Geometry: final body of the model. Coordinates: model frame, mm. A direction names the side the tool comes from. Coordinates: 2 decimals unless noted, no trailing zeros. Write each loop counter-clockwise with the first axis right and the second up, starting at its lowest first coordinate (ties: lowest second). Pieces come first, ordered by that corner, then holes. Notation, with made-up numbers: (57.5, -29.5) - (70.5, -29.5) arc R22 cw to (70.5, -0.5) - close; hole circle Ø1 at (82, 19). An arc over 180 degrees is marked (long way). Answer as a JSON object with one key per item and string values. Group by question number.
Item 1: Line query: line 1 along Y through (x, z) = (25.5, 2.75); line 2 along Y through (x, z) = (51, 6); line 3 along X through (y, z) = (-9, 2.75). Output: solid intervals per line, ascending. Write a range as from..to.
Item 2: Mould query, pull axis X, two halves, no side actions, for faces 5 (the flat face through (7, 46.373, 1)), 6 (the flat face through (73.128, 3, 2)), 7 (the flat face through (2, -44, 0)), 8 (the flat face through (9, -47.627, 5)). Classes: pulls with the +X half, pulls with the -X half, needs draft (parallel to the pull), parting line crosses it, or undercut.
Item 3: First-contact query: pin 1 Ø8 at (x, y) = (54, -39) entering from +Z; pin 2 Ø3 at (y, z) = (5, 5.5) entering from +X. Flat tips, straight axial feed; report the tip coordinate or a pass-through.
Item 4: Set-up query: faces 1 (the flat face through (7, 54.373, 3)), 2 (the flat face through (71.128, -45, 5)), 3 (the flat face through (8, 52.373, 5)), 4 (the flat face through (8, -41.627, 1)). Return all of +Z, -Z, +X, -X, +Y, -Y with unobstructed straight access to the full face (end or side cutting, diameter ignored); none if empty.
Item 5: Section A-A on y = 25.5. Return loops of the section in (x, z).
Item 6: Section B-B on x = 18. Return loops of the section in (y, z).
Item 7: Section C-C on z = 1.25. Return loops of the section in (x, y), and give its area (3 significant figures).
Autodesk Fusion 360 part; units mm, degrees
sketch "Sketch2" plane through (0, 0, 0) normal (0, 0, 1) x (1, 0, 0)
  line L0 (-55.8718, 52.373) -> (71.1282, 52.373)
  line L1 (71.1282, 52.373) -> (71.1282, -47.627)
  line L2 (71.1282, -47.627) -> (-55.8718, -47.627)
  line L3 (-55.8718, -47.627) -> (-55.8718, 52.373)
  line L4 (-51.3718, 46.373) -> (66.6282, 46.373)
  line L5 (66.6282, 46.373) -> (66.6282, -41.627)
  line L6 (66.6282, -41.627) -> (-51.3718, -41.627)
  line L7 (-51.3718, -41.627) -> (-51.3718, 46.373)
  line L8 (-57.8718, 54.373) -> (73.1282, 54.373)
  line L9 (73.1282, 54.373) -> (73.1282, -49.627)
  line L10 (73.1282, -49.627) -> (-57.8718, -49.627)
  line L11 (-57.8718, -49.627) -> (-57.8718, 54.373)
  dimension "d1" = 127
  dimension "d2" = 100
  dimension "d3" = 118
  dimension "d4" = 88
  dimension "d5" = 131
  dimension "d6" = 104
  dimension "d7" = 2
  dimension "d8" = 2
  dimension "d43" = 4.5
  dimension "d44" = 6
extrude "Extrude7" add sketch "Sketch2" along normal blind 3 contours L0 L1 L2 L3
extrude "Extrude8" add sketch "Sketch2" along normal blind 7 contours L8 L9 L10 L11
sketch "Sketch9" plane through (0, 0, 7) normal (0, 0, 1) x (-1, 0, 0)
  line L0 (-71.1282, 47.627) -> (55.8718, 47.627)
  line L1 (55.8718, 47.627) -> (55.8718, -52.373)
  line L2 (55.8718, -52.373) -> (-71.1282, -52.373)
  line L3 (-71.1282, -52.373) -> (-71.1282, 47.627)
  line L4 (57.8718, 49.627) -> (-73.1282, 49.627)
  line L5 (-73.1282, 49.627) -> (-73.1282, -54.373)
  line L6 (-73.1282, -54.373) -> (57.8718, -54.373)
  line L7 (57.8718, -54.373) -> (57.8718, 49.627)
  line L8 (-71.1282, -52.373) -> (-73.1282, -52.373)
  line L9 (-73.1282, -52.373) -> (-73.1282, 42.627)
  line L10 (-73.1282, 42.627) -> (-71.1282, 42.627)
  line L11 (-71.1282, 42.627) -> (-71.1282, -52.373)
  dimension "d39" = 95
extrude "Extrude9" cut sketch "Sketch9" against normal blind 4 contours L3 L5 L8 L9 L10 L11
Checks:
{
 "1": {"line 1": "-49.63..-41.63, 46.37..54.37", "line 2": "-49.63..-47.63, 52.37..54.37", "line 3": "-57.87..-51.37, 66.63..73.13"},
 "2": {"face 5": "undercut", "face 6": "pulls with the +X half", "face 7": "needs draft", "face 8": "undercut"},
 "3": {"pin 1": "z = 3", "pin 2": "x = -55.87"},
 "4": {"face 1": "+Z, -Z, +X, -X, +Y", "face 2": "+Z", "face 3": "+Z, +X", "face 4": "+Z, -Z"},
 "5": {"outline": "(-57.87, 0) - (-51.37, 0) - (-51.37, 3) - (-55.87, 3) - (-55.87, 7) - (-57.87, 7) - close; (66.63, 0) - (73.13, 0) - (73.13, 3) - (66.63, 3) - close"},
 "6": {"outline": "(-49.63, 0) - (-41.63, 0) - (-41.63, 3) - (-47.63, 3) - (-47.63, 7) - (-49.63, 7) - close; (46.37, 0) - (54.37, 0) - (54.37, 7) - (52.37, 7) - (52.37, 3) - (46.37, 3) - close"},
 "7": {"outline": "(-57.87, -49.63) - (73.13, -49.63) - (73.13, 54.37) - (-57.87, 54.37) - close; hole (-51.37, -41.63) - (66.63, -41.63) - (66.63, 46.37) - (-51.37, 46.37) - close", "area": "3,240 mm^2"}
}
